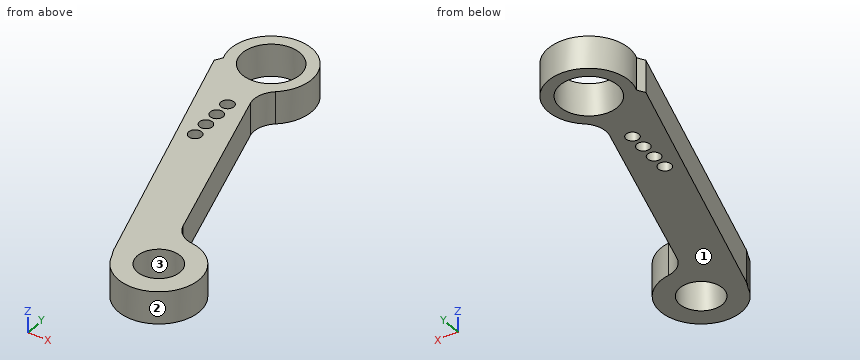
```python
from build123d import *

# Parameters (mm, degrees)
SKETCH1_R           = 2.6375
SKETCH1_R_2         = 3.55
SKETCH1_R_3         = 0.8
BOSS_EXTRUDE1_DEPTH = 4


with BuildPart() as part:
    # Sketch1 → Boss-Extrude1 (new body)
    with BuildSketch(Plane.XY.offset(4)):
        with BuildLine():
            Line((4.361186649, 84.509770663), (3.838692378, 83.622901822))
            Line((3.838692378, 83.622901822), (15.011053362, 49.830662375))
            Line((15.011053362, 49.830662375), (15.45509163, 48.928599175))
            ThreePointArc((15.45509163, 48.928599175), (24.07294723, 47.365734356), (20.790472779, 55.485792426))
            ThreePointArc((20.790472779, 55.485792426), (19.237477826, 56.151424967), (18.290512878, 57.550752445))
            Line((18.290512878, 57.550752445), (11.299825408, 79.414245507))
            ThreePointArc((11.299825408, 79.414245507), (11.27305415, 81.153168904), (12.215576399, 82.614751297))
            ThreePointArc((12.215576399, 82.614751297), (10.152046635, 91.286695043), (4.361186649, 84.509770663))
        make_face()
        with Locations((20.194596002, 50.521426317)):
            Circle(SKETCH1_R, mode=Mode.SUBTRACT)
        with Locations((8.979351439, 86.426161535)):
            Circle(SKETCH1_R_2, mode=Mode.SUBTRACT)
        with Locations((9.4943608, 77.941777919)):
            Circle(SKETCH1_R_3, mode=Mode.SUBTRACT)
        with Locations((9.621598406, 75.845636084)):
            Circle(SKETCH1_R_3, mode=Mode.SUBTRACT)
        with Locations((9.748836013, 73.749494249)):
            Circle(SKETCH1_R_3, mode=Mode.SUBTRACT)
        with Locations((9.87607362, 71.653352414)):
            Circle(SKETCH1_R_3, mode=Mode.SUBTRACT)
    extrude(amount=-BOSS_EXTRUDE1_DEPTH)


solid = part.part
```
Verification items for the finished model (mm, model axes). Face numbers are marked on the shaded views. Round coordinates to 2 decimals unless told otherwise and drop trailing zeros. Order: outer loops, then holes, each group sorted by start corner. A loop starts at its lowest first (then second) coordinate and runs counter-clockwise, first axis right, second up.
1) Cross-section at C-C, the plane y = 88. Record the cut outline in (x, z).
Geometry says:
outline: (4.23, 0) - (5.8, 0) - (5.8, 4) - (4.23, 4) - close; (12.16, 0) - (13.73, 0) - (13.73, 4) - (12.16, 4) - close
2) Depth check by flat-ended pin: pin 1 (1.8 mm diameter, centred on x = 9.49, y = 77.94, fed in from -Z); pin 2 (2 mm diameter, centred on y = 63.5, z = 3, fed in from +X); pin 3 (1.5 mm diameter, centred on y = 54, z = 2, fed in from -X); pin 4 (1 mm diameter, centred on y = 80, z = 2.5, fed in from +X). Enter the tip coordinate at first touch or a pass-through.
Geometry says:
pin 1: stops at z = 0
pin 2: stops at x = 16.71
pin 3: stops at x = 13.38
pin 4: stops at x = 11.27
3) Cross-section at A-A, the plane x = 8. Record the cut outline in (y, z), plus the area to 3 significant figures.
Geometry says:
outline: (71.04, 0) - (83.01, 0) - (83.01, 4) - (71.04, 4) - close; (89.84, 0) - (91.33, 0) - (91.33, 4) - (89.84, 4) - close
area: 53.9 mm2
4) Cross-section at B-B, the plane z = 3. Give the number of separate pieces and of enclosed holes in the cut face, plus the area to 3 significant figures.
Geometry says:
separate pieces: 1
enclosed holes: 6
area: 260 mm2
5) Material ranges on line 1 (Y direction, x = 19.5, z = 2.45); line 2 (X direction, y = 78, z = 2.7); line 3 (X direction, y = 50, z = 3), recorded low to high.
Geometry says:
line 1: y = 45.57 to 47.98, 53.07 to 55.96
line 2: x = 5.7 to 8.7, 10.29 to 11.75
line 3: x = 14.96 to 17.61, 22.78 to 25.17
6) Draft check along X on the marked faces 1, 2 and 3. Enter one of: +X half, -X half, draft (parallel to the pull), parting line (faces both ways), or undercut.
Geometry says:
face 1: draft
face 2: parting line
face 3: undercut
7) Cross-section at D-D, the plane y = 58. Record the cut outline in (x, z), plus the area to 3 significant figures.
Geometry says:
outline: (12.31, 0) - (18.15, 0) - (18.15, 4) - (12.31, 4) - close
area: 23.3 mm2
